Model file for the job. Use its own axes, mm. A direction names the side the tool comes from. Give positions to 0.01 mm unless a question says otherwise; leave off trailing zeros. Order: outer loops, then holes, each group sorted by start corner. A loop starts at its lowest first (then second) coordinate and runs counter-clockwise, first axis right, second up. Notation, with made-up numbers: (-33.75, -10) -> (-26.75, -10) arc R14 cw to (-26.75, 9) -> close; hole circle Ø6 at (19, 51.5). An arc over 180 degrees is marked (long way). Use CSV: the item, a comma, the result in double quotes. Start each with the question number.
1. Cut at A-A on y = 9.5. List the corners of the cut face in (x, z), then the cut area to 3 significant figures.
2. Pull direction X, two halves, no side cores. Call faces 3 (the cylindrical face through (-0.45, 12.64, 1.43)), 4 (the flat face through (0, 0, 0)), 5 (the flat face through (0, 13, 0.75)): released by +X, released by -X, zero draft, split by the parting line, or undercut.
3. Wall check: line 1 (Y direction, x = -0.65, z = -0.75); line 2 (X direction, y = 9.5, z = 0.45). Give the ranges that are in metal, low to high. Write a range as from..to.
4. 3-axis set-ups, long thin cutter, end or side, ignore diameter. For faces 1 (the flat face through (0, 13, -0.75)), 2 (the cylindrical face through (-0.24, 6.006, 0.763)): which of +Z, -Z, +X, -X, +Y, -Y reach the whole face in a straight line?
5. Drop a flat-ended pin along its axis: pin 1 (1 mm diameter, centred on y = 2, z = -0.5, fed in from +X). Give the stop position or say it passes through.
```python
from build123d import *

# Parameters (mm, degrees)
CUT_EXTRUDE2_DEPTH = 13.038376149


with BuildPart() as part:
    # Sketch1 → Revolve1 (revolve)
    with BuildSketch(Plane(origin=(0, 0, 0), x_dir=(0, 0, -1), z_dir=(1, 0, 0)), mode=Mode.PRIVATE) as revolve1_sk:
        with BuildLine():
            ThreePointArc((0.8, 11.7), (0.843933983, 11.806066017), (0.95, 11.85))
            Line((0.95, 11.85), (1.35, 11.85))
            ThreePointArc((1.35, 11.85), (1.456066017, 11.893933983), (1.5, 12))
            Line((1.5, 12), (1.5, 13.268095132))
            ThreePointArc((1.5, 13.268095132), (1.485949045, 13.331481701), (1.446428571, 13.382993046))
            ThreePointArc((1.446428571, 13.382993046), (1.296031396, 13.469838548), (1.125, 13.5))
            Line((1.125, 13.5), (0.917132034, 13.5))
            ThreePointArc((0.917132034, 13.5), (0.895850747, 13.498482682), (0.875, 13.493961424))
            Line((0.875, 13.493961424), (0.875, 12.256185485))
            ThreePointArc((0.875, 12.256185485), (0.845317103, 12.166609847), (0.768016069, 12.112485736))
            ThreePointArc((0.768016069, 12.112485736), (0.646674627, 12.079247272), (0.523906049, 12.051744226))
            ThreePointArc((0.523906049, 12.051744226), (0.263227569, 12.012967451), (0, 12))
            Line((0, 12), (0, 0))
            Line((0, 0), (0.65, 0))
            Line((0.65, 0), (0.8, 0.15))
            Line((0.8, 0.15), (0.8, 11.7))
        make_face()
    revolve(revolve1_sk.sketch.rotate(Axis((0, 13.5, 0), (0, -1, 0)), 180), axis=Axis((0, 13.5, 0), (0, -1, 0)))


with BuildPart() as body_2:
    # Sketch1_3 → Revolve2 (revolve)
    with BuildSketch(Plane(origin=(0, 0, 0), x_dir=(0, 0, -1), z_dir=(1, 0, 0)), mode=Mode.PRIVATE) as revolve2_sk:
        with BuildLine():
            ThreePointArc((0.725, 12.29691396), (0.668295774, 12.138368245), (0.523906049, 12.051744226))
            ThreePointArc((0.523906049, 12.051744226), (0.646674627, 12.079247272), (0.768016069, 12.112485736))
            ThreePointArc((0.768016069, 12.112485736), (0.845317103, 12.166609847), (0.875, 12.256185485))
            Line((0.875, 12.256185485), (0.875, 13.493961424))
            ThreePointArc((0.875, 13.493961424), (0.840648826, 13.479036115), (0.811066017, 13.456066017))
            Line((0.811066017, 13.456066017), (0.725, 13.37))
            Line((0.725, 13.37), (0.725, 12.29691396))
        make_face()
    revolve(revolve2_sk.sketch.rotate(Axis((0, 13.5, 0), (0, -1, 0)), 180), axis=Axis((0, 13.5, 0), (0, -1, 0)))

    # Sketch2 → Cut-Extrude2 (cut, through all)
    with BuildSketch(Plane.XZ.offset(-11.85)):
        Polygon((-0.433012702, 0.75), (-0.866025404, 0), (-0.433012702, -0.75), (0.433012702, -0.75), (0.866025404, 0), (0.433012702, 0.75), align=None)
    extrude(amount=-CUT_EXTRUDE2_DEPTH, mode=Mode.SUBTRACT)


with BuildPart() as part_1:
    add(part.part)

    # Combine1: union body 2
    add(body_2.part)


solid = part_1.part
```
Verdict:
1,outline,"circle Ø1.6 at (0, 0)"
1,area,"2.01 mm^2"
2,face 3,"split by the parting line"
2,face 4,"zero draft"
2,face 5,"undercut"
3,line 1,"11.85..13.5"
3,line 2,"-0.66..0.66"
4,face 1,"+Y"
4,face 2,"-Y"
5,pin 1,"x = 0.8"
